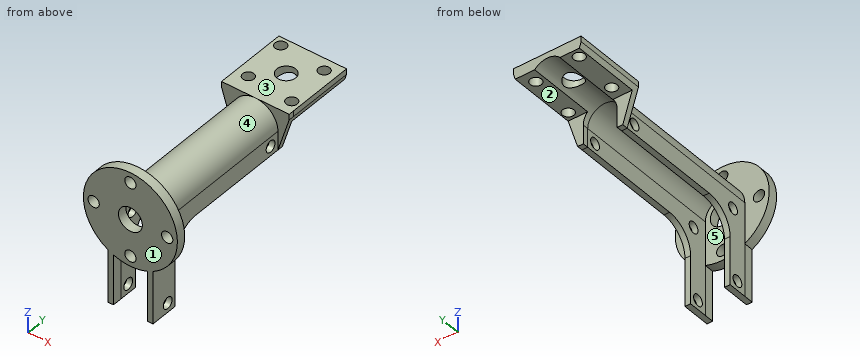
```python
from build123d import *

# Parameters (mm, degrees)
SKETCH_R        = 1.5
SKETCH_R_2      = 2.5
PAD_DEPTH       = 3
PAD001_DEPTH    = 1.5
PAD002_DEPTH    = 40
SKETCH005_R     = 1.5
POCKET_DEPTH    = 13
POCKET001_DEPTH = 25
POCKET002_DEPTH = 25
SKETCH007_R     = 3.175
SKETCH007_R_2   = 1.5
PAD003_DEPTH    = 2.5


with BuildPart() as part:
    # Sketch → Pad (new body)
    with BuildSketch(Plane.XY):
        Polygon((0, 0), (18, 0), (18, 18), (0, 18), (0, 10.5), (0, 7.5), align=None)
        with Locations((2.2824855787, 15.7175144213)):
            Circle(SKETCH_R, mode=Mode.SUBTRACT)
        with Locations((14.6568542495, 14.6568542495)):
            Circle(SKETCH_R, mode=Mode.SUBTRACT)
        with Locations((3.3431457505, 3.3431457505)):
            Circle(SKETCH_R, mode=Mode.SUBTRACT)
        with Locations((15.7175144213, 2.2824855787)):
            Circle(SKETCH_R, mode=Mode.SUBTRACT)
        with Locations((9, 9)):
            Circle(SKETCH_R_2, mode=Mode.SUBTRACT)
    extrude(amount=PAD_DEPTH)

    # Sketch002 → Pad001 (new body)
    with BuildSketch(Plane.XZ):
        Polygon((0, 3), (18, 3), (17.9999999631, -7.9988470638), (0, -8), align=None)
    extrude(amount=PAD001_DEPTH)

    # Sketch001 → Pad002 (new body)
    with BuildSketch(Plane.XZ.offset(1.5)):
        with BuildLine():
            ThreePointArc((13.5, -3), (9, 1.5), (4.5, -3))
            Line((4.5, -3), (4.5001284117, -27.9999999997))
            Line((4.5001284117, -27.9999999997), (3.0001284117, -27.9999999997))
            Line((3.0001284117, -27.9999999997), (3, -3))
            ThreePointArc((15, -3), (9, 3), (3, -3))
            Line((15, -3), (15.0001284117, -27.9999999997))
            Line((15.0001284117, -27.9999999997), (13.5001284117, -27.9999999997))
            Line((13.5001284117, -27.9999999997), (13.5, -3))
        make_face()
    extrude(amount=PAD002_DEPTH)

    # Sketch005 → Pocket (cut)
    with BuildSketch(Plane(origin=(14.9999845902, 0, 7.70469e-05), x_dir=(0, 1, 0), z_dir=(1, 0, 5.1365e-06))):
        with Locations((-4, -5.500077047)):
            Circle(SKETCH005_R)
        with Locations((-37.5, -7.000077047)):
            Circle(SKETCH005_R)
        with Locations((-39, -25.500077047)):
            Circle(SKETCH005_R)
        with BuildLine():
            Line((-36.5, -28.000077047), (-36.4999999999, -15.1369541066))
            ThreePointArc((-29.3631590976, -8.000077047), (-34.4096804325, -10.0904221815), (-36.4999999999, -15.1369541066))
            Line((-29.3631590976, -8.000077047), (-1.4999991941, -8.000077047))
            Line((-1.5, -28.000077047), (-1.4999991941, -8.000077047))
            Line((-36.5, -28.000077047), (-1.5, -28.000077047))
        make_face()
    extrude(amount=-POCKET_DEPTH, mode=Mode.SUBTRACT)

    # Sketch006 → Pocket001 (cut)
    with BuildSketch(Plane.XZ.offset(1.5)):
        Polygon((0, 1.5), (2.9999999938, -7.999807844), (0, -8), align=None)
        Polygon((17.9999999631, -7.9988470638), (14.9999999692, -7.9990392199), (17.999999995, 1.5), align=None)
    extrude(amount=-POCKET001_DEPTH, mode=Mode.SUBTRACT)

    # Sketch008 → Pocket002 (cut)
    with BuildSketch(Plane.XZ.offset(1.5)):
        with BuildLine():
            Line((4.5000000092, -2.9997117644), (4.5000256809, -7.9997117643))
            Line((4.5000256809, -7.9997117643), (13.5000256779, -7.9991352962))
            Line((13.4999999169, -2.9991352963), (13.5000256779, -7.9991352962))
            ThreePointArc((13.4999999169, -2.9991352963), (8.999711766, 1.4999999908), (4.5000000092, -2.9997117644))
        make_face()
    extrude(amount=-POCKET002_DEPTH, mode=Mode.SUBTRACT)

    # Sketch007 → Pad003 (new body)
    with BuildSketch(Plane.XZ.offset(41.5)):
        with BuildLine():
            ThreePointArc((15.0000563256, -13.9658252808), (8.9999357942, 9.4999999998), (3.0000563259, -13.9658869184))
            Line((3.0000563259, -13.9658869184), (3.0001284117, -27.9999999997))
            Line((3.0001284117, -27.9999999997), (4.5001284117, -27.9999999997))
            Line((4.5000599011, -14.6619269037), (4.5001284117, -27.9999999997))
            ThreePointArc((4.5000599011, -14.6619269037), (9.0000642058, -15.4999999998), (13.5000599009, -14.6618806755))
            Line((13.5000599009, -14.6618806755), (13.5001284117, -27.9999999997))
            Line((13.5001284117, -27.9999999997), (15.0001284117, -27.9999999997))
            Line((15.0000563256, -13.9658252808), (15.0001284117, -27.9999999997))
        make_face()
        with Locations((9, -3)):
            Circle(SKETCH007_R, mode=Mode.SUBTRACT)
        with Locations((-0.779, -3)):
            Circle(SKETCH007_R_2, mode=Mode.SUBTRACT)
        with Locations((9, -12.779)):
            Circle(SKETCH007_R_2, mode=Mode.SUBTRACT)
        with Locations((9, 6.779)):
            Circle(SKETCH007_R_2, mode=Mode.SUBTRACT)
        with Locations((18.779, -3)):
            Circle(SKETCH007_R_2, mode=Mode.SUBTRACT)
    extrude(amount=PAD003_DEPTH)


solid = part.part
```
Model file for the job. Use its own axes, mm. Face numbers are marked on the shaded views. A direction names the side the tool comes from. Give positions to 0.01 mm unless a question says otherwise; leave off trailing zeros. Loops run counter-clockwise (first coordinate to the right, second up) from the corner with the lowest first, then second, coordinate; pieces in that order, holes last. Notation, with made-up numbers: (1.5, 27) - (32.5, 27) arc R19 ccw to (32.5, 64) - close; hole circle Ø10 at (-1, 34). An arc over 180 degrees is marked (long way). One line per item, written item: value. Start each with the question number.
1. Pin check, flat tips, straight feed: pin 1 (5 mm diameter, centred on y = -37.5, z = -7, fed in from -X); pin 2 (2.5 mm diameter, centred on y = -37.5, z = -7, fed in from -X); pin 3 (0.5 mm diameter, centred on x = 4, y = -17.5, fed in from -Z); pin 4 (5 mm diameter, centred on x = 2.28, y = 15.72, fed in from -Z). Stop position of each tip, or through.
2. Slice it at B-B (y = -20). List the corners of the cut face in (x, z), plus the area to 3 significant figures.
3. Probe L1, parallel to Z at x = 9, y = -42.25 (3 decimals); L2, parallel to Y at x = 4, z = -25.5; L3, parallel to Y at x = 9, z = 2.25. List the from-to ranges inside material, lowest first. Write a range as from..to.
4. Slice it at A-A (y = -4). List the corners of the cut face in (x, z), plus the area to 3 significant figures.
5. Slice it at C-C (x = -1.5). List the corners of the cut face in (y, z).
6. Pull direction X, two halves, no side cores. Call the marked faces 3, 4 and 5: pulls with the +X half, pulls with the -X half, needs draft (parallel to the pull), parting line crosses it, or undercut.
7. Which spindle directions (+Z, -Z, +X, -X, +Y, -Y) get a long thin tool onto all of the face, cutting with end or side? Do the marked faces 1 and 2. Say none if no direction does.
Solution:
1. pin 1: stops at x = 3
1. pin 2: passes through
1. pin 3: stops at z = -8
1. pin 4: stops at z = 0
2. outline: (3, -8) - (4.5, -8) - (4.5, -3) arc R4.5 cw to (13.5, -3) - (13.5, -8) - (15, -8) - (15, -3) arc R6 ccw to (3, -3) - close
2. area: 39.7 mm^2
3. L1: z = -15.5..-14.279, -11.279..-6.175, 0.175..5.279, 8.279..9.5
3. L2: y = -44..-40.5, -37.5..-36.5
3. L3: y = -44..6.5, 11.5..18
4. outline: (3, -8) - (4.5, -8) - (4.5, -7) - (3, -7) - close; (3, -4) - (4.5, -4) - (4.5, -3) arc R4.5 cw to (13.5, -3) - (13.5, -4) - (15, -4) - (15, -3) arc R6 ccw to (3, -3) - close; (13.5, -8) - (15, -8) - (15, -7) - (13.5, -7) - close
4. area: 30.7 mm^2
5. outline: (-44, -9.78) - (-41.5, -9.78) - (-41.5, -4.32) - (-44, -4.32) - close; (-44, -1.68) - (-41.5, -1.68) - (-41.5, 3.78) - (-44, 3.78) - close
6. face 3: needs draft
6. face 4: parting line crosses it
6. face 5: undercut
7. face 1: +Z, -Z, +X, -X, -Y
7. face 2: -Z, +X, -X, +Y
